from build123d import *

# Parameters (mm, degrees)
SKETCH1_R           = 4
SKETCH1_R_2         = 2.5
BOSS_EXTRUDE2_DEPTH = 3
CUT_EXTRUDE2_REACH  = 186.619
SKETCH2_R           = 4
CUT_EXTRUDE3_REACH  = 186.619
SKETCH3_R           = 2.1


with BuildPart() as part:
    # Sketch1 → Boss-Extrude2 (new body)
    with BuildSketch(Plane(origin=(0, 0, 0), x_dir=(1, 0, 0), z_dir=(0, 1, 0))):
        with BuildLine():
            Line((9.170700563, 3.987261114), (7.876862883, 6.963087778))
            ThreePointArc((7.876862883, 6.963087778), (7.198186925, 12.679447551), (9.783335319, 17.822829502))
            ThreePointArc((9.783335319, 17.822829502), (19.286109016, 34.269627525), (20.356745206, 53.234163146))
            ThreePointArc((20.356745206, 53.234163146), (20.462846426, 57.276901224), (22.161434095, 60.947022282))
            Line((22.161434095, 60.947022282), (43.375248586, 89.614346273))
            ThreePointArc((43.375248586, 89.614346273), (44.111659282, 90.146760278), (45.020325467, 90.156307579))
            ThreePointArc((45.020325467, 90.156307579), (48.577517121, 91.673723777), (47.683482049, 95.43628483))
            ThreePointArc((47.683482049, 95.43628483), (14.052723286, 128.748405766), (-8.766929777, 170.221153086))
            ThreePointArc((-8.766929777, 170.221153086), (-25.192986973, 176.818173889), (-30.319391627, 159.875446429))
            ThreePointArc((-30.319391627, 159.875446429), (-16.336845375, 106.715190551), (-32.562737633, 54.196195652))
            ThreePointArc((-32.562737633, 54.196195652), (-34.453402431, 41.987624374), (-26.539917992, 32.500760293))
            ThreePointArc((-26.539917992, 32.500760293), (-13.161486595, 19.643005303), (-9.904938494, 1.37557022))
            ThreePointArc((-9.904938494, 1.37557022), (1.356469191, -9.907572424), (9.170700563, 3.987261114))
        make_face()
        with Locations(Location((0, 0, 0), (0, 0, 270))):
            Circle(SKETCH1_R, mode=Mode.SUBTRACT)
        with Locations(Location((-20, 46, 0), (0, 0, 270))):
            Circle(SKETCH1_R_2, mode=Mode.SUBTRACT)
    extrude(amount=BOSS_EXTRUDE2_DEPTH)

    # Sketch2 → Cut-Extrude2 (cut, up to next)
    with BuildSketch(Plane(origin=(0, 3, 0), x_dir=(1, 0, 0), z_dir=(0, 1, 0)), mode=Mode.PRIVATE) as cut_extrude2_sk1:
        with Locations(Location((-20, 166, 0), (0, 0, 270))):
            Circle(SKETCH2_R)
    cut_extrude2_tool1 = extrude(cut_extrude2_sk1.sketch, amount=-CUT_EXTRUDE2_REACH, mode=Mode.PRIVATE) & part.part
    # Sketch2 → Cut-Extrude2 (cut, up to next)
    with BuildSketch(Plane(origin=(0, 3, 0), x_dir=(1, 0, 0), z_dir=(0, 1, 0)), mode=Mode.PRIVATE) as cut_extrude2_sk2:
        with BuildLine():
            Line((24.08650635, 90.617794829), (-1.761817511, 71.71243196))
            ThreePointArc((-1.761817511, 71.71243196), (-5.273300355, 71.690348613), (-6.400182005, 75.01617741))
            ThreePointArc((-6.400182005, 75.01617741), (-2.152471882, 94.978495294), (-1.500425627, 115.37731909))
            ThreePointArc((-1.500425627, 115.37731909), (0.438343778, 118.355781743), (3.85956825, 117.393861946))
            ThreePointArc((3.85956825, 117.393861946), (13.636229053, 105.89490145), (24.339781746, 95.253325031))
            ThreePointArc((24.339781746, 95.253325031), (25.310999303, 92.875575481), (24.08650635, 90.617794829))
        make_face()
    cut_extrude2_tool2 = extrude(cut_extrude2_sk2.sketch, amount=-CUT_EXTRUDE2_REACH, mode=Mode.PRIVATE) & part.part
    # Sketch2 → Cut-Extrude2 (cut, up to next)
    with BuildSketch(Plane(origin=(0, 3, 0), x_dir=(1, 0, 0), z_dir=(0, 1, 0)), mode=Mode.PRIVATE) as cut_extrude2_sk3:
        with BuildLine():
            Line((1.399941693, 47.961192116), (-7.607238393, 42.3183015))
            ThreePointArc((-7.607238393, 42.3183015), (-8.997062251, 40.099202055), (-8.114849087, 37.633900322))
            ThreePointArc((-8.114849087, 37.633900322), (-5.481535576, 34.820910528), (-3.098522666, 31.792957242))
            ThreePointArc((-3.098522666, 31.792957242), (-0.586190052, 30.546672377), (1.858342535, 31.921191043))
            ThreePointArc((1.858342535, 31.921191043), (4.848412053, 38.347783431), (5.991700338, 45.343103105))
            ThreePointArc((5.991700338, 45.343103105), (4.478604072, 48.025038621), (1.399941693, 47.961192116))
        make_face()
    cut_extrude2_tool3 = extrude(cut_extrude2_sk3.sketch, amount=-CUT_EXTRUDE2_REACH, mode=Mode.PRIVATE) & part.part
    add(cut_extrude2_tool1.solids().sort_by_distance((-20, 3, -166))[0], mode=Mode.SUBTRACT)
    add(cut_extrude2_tool2.solids().sort_by_distance((6.92649, 3, -93.946856))[0], mode=Mode.SUBTRACT)
    add(cut_extrude2_tool3.solids().sort_by_distance((-0.710411, 3, -39.721946))[0], mode=Mode.SUBTRACT)

    # Sketch3 → Cut-Extrude3 (cut, up to next)
    with BuildSketch(Plane(origin=(0, 3, 0), x_dir=(1, 0, 0), z_dir=(0, 1, 0)), mode=Mode.PRIVATE) as cut_extrude3_sk1:
        with Locations(Location((2.309703224, 131.433631836, 0), (0, 0, 270))):
            Circle(SKETCH3_R)
    cut_extrude3_tool1 = extrude(cut_extrude3_sk1.sketch, amount=-CUT_EXTRUDE3_REACH, mode=Mode.PRIVATE) & part.part
    # Sketch3 → Cut-Extrude3 (cut, up to next)
    with BuildSketch(Plane(origin=(0, 3, 0), x_dir=(1, 0, 0), z_dir=(0, 1, 0)), mode=Mode.PRIVATE) as cut_extrude3_sk2:
        with Locations(Location((34.609964816, 95.56055708, 0), (0, 0, 270))):
            Circle(SKETCH3_R)
    cut_extrude3_tool2 = extrude(cut_extrude3_sk2.sketch, amount=-CUT_EXTRUDE3_REACH, mode=Mode.PRIVATE) & part.part
    # Sketch3 → Cut-Extrude3 (cut, up to next)
    with BuildSketch(Plane(origin=(0, 3, 0), x_dir=(1, 0, 0), z_dir=(0, 1, 0)), mode=Mode.PRIVATE) as cut_extrude3_sk3:
        with Locations(Location((17.205589144, 112.367767299, 0), (0, 0, 270))):
            Circle(SKETCH3_R)
    cut_extrude3_tool3 = extrude(cut_extrude3_sk3.sketch, amount=-CUT_EXTRUDE3_REACH, mode=Mode.PRIVATE) & part.part
    add(cut_extrude3_tool1.solids().sort_by_distance((2.309703, 3, -131.433632))[0], mode=Mode.SUBTRACT)
    add(cut_extrude3_tool2.solids().sort_by_distance((34.609965, 3, -95.560557))[0], mode=Mode.SUBTRACT)
    add(cut_extrude3_tool3.solids().sort_by_distance((17.205589, 3, -112.367767))[0], mode=Mode.SUBTRACT)


solid = part.part
Work out the finished part from the listing and answer in its coordinate system (mm). A direction names the side the tool comes from. Give positions to 0.01 mm unless a question says otherwise; leave off trailing zeros. Loops run counter-clockwise (first coordinate to the right, second up) from the corner with the lowest first, then second, coordinate; pieces in that order, holes last. Notation, with made-up numbers: (6.25, 7.5) - (37.25, 7.5) arc R25 cw to (37.25, 39.5) - close; hole circle Ø5 at (29.25, 7). An arc over 180 degrees is marked (long way). Answer in a Markdown table with one row per item.
(1) Section A-A (z = -166) is taken. Give the vertices of the cut face in (x, y).
Results list:
| item | result |
|---|---|
| outline | (-32, 0) - (-24, 0) - (-24, 3) - (-32, 3) - close; (-16, 0) - (-7.11, 0) - (-7.11, 3) - (-16, 3) - close |
(2) Section B-B (y = 2.4) is taken. State how many separate pieces and enclosed holes the cut face has, and give its area (3 significant figures).
Results list:
| item | result |
|---|---|
| separate pieces | 1 |
| enclosed holes | 8 |
| area | 6,120 mm² |
(3) Section D-D (z = -136) is taken. Give the vertices of the cut face in (x, y).
Results list:
| item | result |
|---|---|
| outline | (-20.07, 0) - (8.88, 0) - (8.88, 3) - (-20.07, 3) - close |
(4) Consider L1, parallel to X at y = 2, z = 0; L2, parallel to X at y = 1.4, z = -114; L3, parallel to Z at x = 24.5, y = 2.6. Determine where each line is inside the solid, lowest interval first. Write a range as [from, to].
Results list:
| item | result |
|---|---|
| L1 | x = [-10, -4], [4, 10] |
| L2 | x = [-16.45, -1.43], [6.58, 15.88], [18.53, 26.61] |
| L3 | z = [-116.24, -95.1], [-90.98, -64.11] |
(5) Flat-ended cylindrical pins translate along their axes: pin 1 Ø1.5 at (x, y) = (-16, 1.5) entering from -Z; pin 2 Ø3.5 at (x, z) = (2.31, -131.43) entering from -Y. Find the tip coordinate at first contact, or state that the pin passes through.
Results list:
| item | result |
|---|---|
| pin 1 | stops at z = -177.55 |
| pin 2 | passes through |
(6) A tool of negligible diameter and unlimited length cuts with its end or side. For faces 1 (the face through (4.82, 1.52, -38.25)), 2 (the face through (-12, 3, -85)), from which of +Z, -Z, +X, -X, +Y, -Y can it reach the whole face along a straight path? Write none if from no direction.
Results list:
| item | result |
|---|---|
| face 1 | +Y, -Y |
| face 2 | +Z, -Z, +X, -X, +Y |
(7) Section C-C (x = -20) is taken. Give the vertices of the cut face in (y, z), and give its area (3 significant figures).
Results list:
| item | result |
|---|---|
| outline | (0, -178) - (3, -178) - (3, -170) - (0, -170) - close; (0, -162) - (3, -162) - (3, -135.74) - (0, -135.74) - close; (0, -81.94) - (3, -81.94) - (3, -48.5) - (0, -48.5) - close; (0, -43.5) - (3, -43.5) - (3, -28.2) - (0, -28.2) - close |
| area | 249 mm² |
(8) For a pull along Z with two mould halves and no side action, classify faces 3 (the face through (-3.04, 1.52, -45.18)), 4 (the face through (-12, 0, -85)), 5 (the face through (14.454, 1.479, -128.218)) as pulls with the +Z half, pulls with the -Z half, needs draft (parallel to the pull), parting line crosses it, or undercut.
Results list:
| item | result |
|---|---|
| face 3 | undercut |
| face 4 | needs draft |
| face 5 | pulls with the -Z half |
